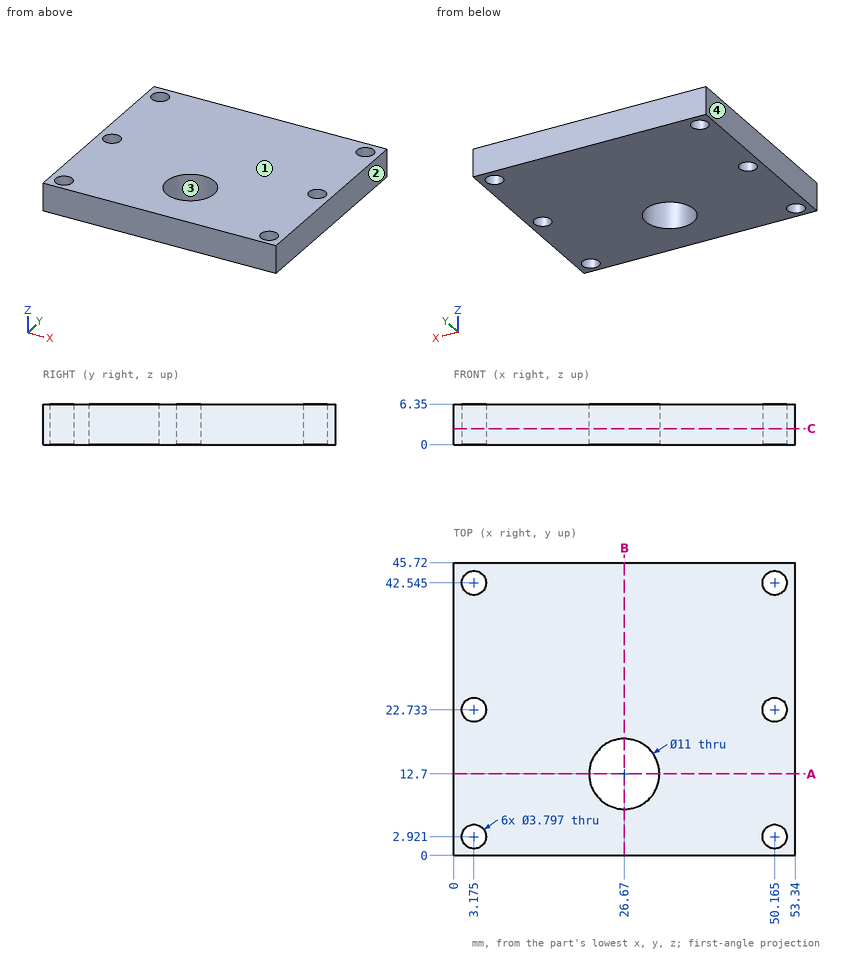
Answer from the drawing. Dimensions are ordinates in mm from the lowest x, y and z of the part. Give positions to 0.01 mm unless a question says otherwise; leave off trailing zeros. Write each loop counter-clockwise with the first axis right and the second up, starting at its lowest first coordinate (ties: lowest second). Pieces come first, ordered by that corner, then holes. Notation, with made-up numbers: M 7.25,-19.75 L 32.25,-19.75 A12 ccw 32.25,-7.75 Z; hole C 5,12 d3. An arc over 180 degrees is marked long. Answer as CSV lines item,"result".
Q1. A cutting plane is placed at C-C on z = 2.5. Write down the section's boundary in (x, y) (1 decimal).
A:
outline,"M 0,0 L 53.3,0 L 53.3,45.7 L 0,45.7 Z; hole C 3.2,2.9 d3.8; hole C 3.2,22.7 d3.8; hole C 3.2,42.5 d3.8; hole C 26.7,12.7 d11; hole C 50.2,2.9 d3.8; hole C 50.2,22.7 d3.8; hole C 50.2,42.5 d3.8"
Q2. Find the intervals of material crossed by probe 1 along X at (y, z) = (21, 6); probe 2 along X at (y, z) = (42, 4.5); probe 3 along Y at (x, z) = (26.67, 3.5), in increasing order. Write a range as [from, to].
A:
probe 1,"x = [0, 2.4], [3.95, 49.39], [50.94, 53.34]"
probe 2,"x = [0, 1.36], [4.99, 48.35], [51.98, 53.34]"
probe 3,"y = [0, 7.2], [18.2, 45.72]"
Q3. A cutting plane is placed at A-A on y = 12.7. Write down the section's boundary in (x, z), plus the area to 3 significant figures.
A:
outline,"M 0,0 L 21.17,0 L 21.17,6.35 L 0,6.35 Z; M 32.17,0 L 53.34,0 L 53.34,6.35 L 32.17,6.35 Z"
area,"269 mm²"
Q4. A cutting plane is placed at B-B on x = 26.67. Write down the section's boundary in (y, z).
A:
outline,"M 0,0 L 7.2,0 L 7.2,6.35 L 0,6.35 Z; M 18.2,0 L 45.72,0 L 45.72,6.35 L 18.2,6.35 Z"
Q5. The mould has two halves that part along X. Classify the marked faces 1, 2, 3 and 4: +X half, -X half, draft (parallel to the pull), parting line (faces both ways), or undercut.
A:
face 1,"draft"
face 2,"+X half"
face 3,"undercut"
face 4,"-X half"
